Source: CAD feature listing. Evaluate the final solid. Frame: model axes, mm. Give positions to 0.01 mm unless a question says otherwise; leave off trailing zeros. Write each loop counter-clockwise with the first axis right and the second up, starting at its lowest first coordinate (ties: lowest second). Pieces come first, ordered by that corner, then holes. Notation, with made-up numbers: (47.5, 17) - (77.5, 17) arc R31 cw to (77.5, 52) - close; hole circle Ø11 at (76.25, 19). An arc over 180 degrees is marked (long way). Answer as a JSON object with one key per item and string values. Group by question number.
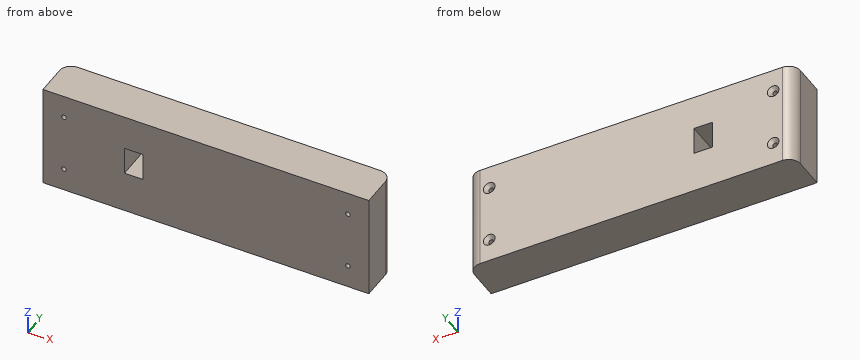
Autodesk Inventor part; units mm, degrees
ref_plane "YZ Plane" through (0, 0, 0) normal (1, 0, 0) x (0, 1, 0)
ref_plane "XZ Plane" through (0, 0, 0) normal (0, 1, 0) x (-1, 0, 0)
ref_plane "XY Plane" through (0, 0, 0) normal (0, 0, 1) x (1, 0, 0)
sketch "Skizze1" plane through (0, 0, 0) normal (0, 1, 0) x (-1, 0, 0)
  line L0 (0, 0) -> (140, 0)
  line L1 (140, 0) -> (140, -45)
  line L2 (140, -45) -> (0, -45)
  line L3 (0, -45) -> (0, 0)
  dimension "d0" = 140
  dimension "d1" = 45
extrude "Extrusion1" add sketch "Skizze1" along normal blind 18
sketch "Skizze2" plane through (0, 18, 0) normal (0, 1, 0) x (1, 0, 0)
  line L0 (0, 0) -> (0, 45)
  line L1 (0, 45) -> (-140, 45)
  line L2 (-140, 45) -> (-140, 0)
  point P0 (-131, 35)
  point P1 (-131, 10)
  point P2 (-9, 35)
  point P3 (-9, 10)
  dimension "d14" = 10
  dimension "d15" = 25
  dimension "d16" = 10
  dimension "d17" = 25
  dimension "d18" = 9
  dimension "d19" = 9
hole "Bohrung1" at (-131, 18, -35) at (-131, 18, -10) at (-9, 18, -35) at (-9, 18, -10) direction (0, -1, 0) diameter 2 end through all countersink diameter 5 countersink angle 90
fillet "Rundung3" radius 5 2 edges at (0, 18, -22.5) (-140, 18, -22.5)
sketch "Skizze3" plane through (0, 18, 0) normal (0, 1, 0) x (1, 0, 0)
  line L0 (-135, 0) -> (-5, 0)
  line L1 (-97, 15) -> (-105, 15)
  line L2 (-105, 15) -> (-105, 27)
  line L3 (-105, 27) -> (-97, 27)
  line L4 (-97, 27) -> (-97, 15)
  line L5 (0, 0) -> (0, 45)
  line L6 (-140, 45) -> (-140, 0)
  dimension "d32" = 8
  dimension "d33" = 12
  dimension "d34" = 15
  dimension "d36" = 35
extrude "Extrusion2" cut sketch "Skizze3" against normal blind 18
sketch "Skizze4" plane through (-140, 0, 0) normal (0, 0, 1) x (1, 0, 0)
  point P0 (131, 3)
properties part number "Seitenteil_mit_schalter" material "Eiche, weiß"
Q1. First-contact query: pin 1 Ø2.5 at (x, z) = (-9, -10) entering from +Y; pin 2 Ø1.8 at (x, z) = (-131, -10) entering from +Y; pin 3 Ø5 at (y, z) = (16, -33) entering from +X. Flat tips, straight axial feed; report the tip coordinate or a pass-through.
Q2. Section B-B on y = 11.75. Return the cut outline in (x, z).
Q3. Section A-A on z = -16.5. Return the cut outline in (x, y).
Q4. Ray query, probe 1 along Z at (x, y) = (-9, 5); probe 2 along X at (y, z) = (4.25, -35); probe 3 along X at (y, z) = (11, -16). Return the intervals inside material, ascending. Write a range as [from, to].
Taken from the geometry:
{
 "1": {"pin 1": "stops at y = 16.75", "pin 2": "passes through", "pin 3": "stops at x = -0.03"},
 "2": {"outline": "(-140, -45) - (0, -45) - (0, 0) - (-140, 0) - close; hole circle Ø2 at (-131, -35); hole circle Ø2 at (-131, -10); hole (-105, -27) - (-97, -27) - (-97, -15) - (-105, -15) - close; hole circle Ø2 at (-9, -35); hole circle Ø2 at (-9, -10)"},
 "3": {"outline": "(-140, 0) - (-105, 0) - (-105, 18) - (-135, 18) arc R5 ccw to (-140, 13) - close; (-97, 0) - (0, 0) - (0, 13) arc R5 ccw to (-5, 18) - (-97, 18) - close"},
 "4": {"probe 1": "z = [-45, -36], [-34, -11], [-9, 0]", "probe 2": "x = [-140, -132], [-130, -10], [-8, 0]", "probe 3": "x = [-140, -105], [-97, 0]"}
}
